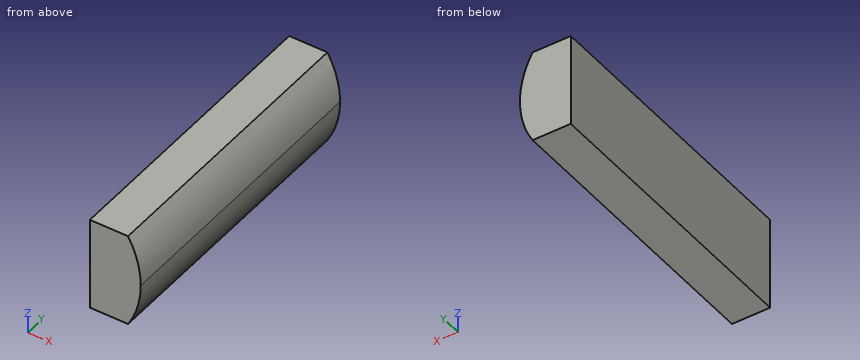
from build123d import *

# Parameters (mm, degrees)
F1_DEPTH = 345


with BuildPart() as f1:
    # F0 (on Front) → F1 (new body)
    with BuildSketch(Plane.XZ):
        with BuildLine():
            Line((0, 110), (0, 55))
            Line((0, 55), (60, 55))
            ThreePointArc((60, 55), (56.182747, 83.504386), (45, 110))
            Line((45, 110), (0, 110))
        make_face()
        with BuildLine():
            Line((0, 55), (0, 0))
            Line((0, 0), (45, 0))
            ThreePointArc((45, 0), (56.182747, 26.495614), (60, 55))
            Line((60, 55), (0, 55))
        make_face()
    extrude(amount=-F1_DEPTH)


solid = f1.part
Could you check a few things on this model? Use its own coordinates, in mm. Coordinates: 2 decimals unless noted, no trailing zeros. Order: outer loops, then holes, each group sorted by start corner. A loop starts at its lowest first (then second) coordinate and runs counter-clockwise, first axis right, second up. Notation, with made-up numbers: (-35, -23) -> (-10, -23) arc R22 cw to (-10, 4) -> close; hole circle Ø5 at (71, 83). An arc over 180 degrees is marked (long way). One line per item, written item: value. Start each with the question number.
1) I'm going to push flat-ended pins straight in: pin 1 (8 mm diameter, centred on y = 201, z = 67, fed in from -X); pin 2 (1 mm diameter, centred on y = 243, z = 25, fed in from +X). Where does each tip first touch, or does it pass through?
2) If I drill on L1, parallel to X at y = 122, z = 58.5; L2, parallel to X at y = 60.5, z = 53; L3, parallel to Z at x = 51.5, y = 276.5, over which ranges is the centre line in solid material (lowest first)? Write a range as [from, to].
3) Imagine slicing it at B-B on z = 29. List the corners of the cut face in (x, y) for me.
4) Imagine slicing it at A-A on y = 239. List the corners of the cut face in (x, z) for me, plus the area to 3 significant figures.
5) Imagine slicing it at C-C on x = 48. List the corners of the cut face in (y, z) for me.
Answer list:
1. pin 1: stops at x = 0
1. pin 2: stops at x = 55.91
2. L1: x = [0, 59.94]
2. L2: x = [0, 59.98]
2. L3: z = [12.94, 97.06]
3. outline: (0, 0) -> (56.83, 0) -> (56.83, 345) -> (0, 345) -> close
4. outline: (0, 0) -> (45, 0) arc R108.33 ccw to (60, 55) arc R108.33 ccw to (45, 110) -> (0, 110) -> close
4. area: 6,070 mm2
5. outline: (0, 5.44) -> (345, 5.44) -> (345, 104.56) -> (0, 104.56) -> close
